For this review, take the finished solid that the model builds, in its own axes (mm). Face numbers are marked on the shaded views. A direction names the side the tool comes from. Round coordinates to 2 decimals unless told otherwise and drop trailing zeros. Loops run counter-clockwise (first coordinate to the right, second up) from the corner with the lowest first, then second, coordinate; pieces in that order, holes last.
1. Clearance check with flat-ended pins moving along their axes: pin 1 Ø2 at (x, z) = (8.5, 10.5) entering from -Y; pin 2 Ø1 at (y, z) = (-14, 14.5) entering from -X; pin 3 Ø4 at (x, z) = (-12.5, 13) entering from +Y. State where each tip first meets the part, or that it passes through.
2. Tool access review of the marked faces 1, 2 and 3: name each direction out of +Z, -Z, +X, -X, +Y, -Y from which nothing blocks a thin tool from reaching the whole face with its end or side.
3. Consider section C-C on z = 3. State the section outline as (x, y) points, then the cut area to 3 significant figures.
4. Consider section B-B on x = 23.5. State the section outline as (y, z) points, then the cut area to 3 significant figures.
5. Draft analysis for pull direction Y (two halves, no side actions). For the marked faces 4, 5, 6 and 7, state which applies: released by +Y, released by -Y, zero draft, split by the parting line, or undercut.
6. Consider section D-D on x = -8. State the section outline as (y, z) points, then the cut area to 3 significant figures.
7. To check wall thickness, follow line 1 along Y through (x, z) = (-23.5, 3.85); line 2 along Y through (x, z) = (0, 8); line 3 along Z through (x, y) = (-17.5, -22). State the ranges of each line that lie inside material, in increasing order.
8. Consider section A-A on y = 0. State the section outline as (x, z) points.
from build123d import *

# Parameters (mm, degrees)
SKETCH1_W           = 53
SKETCH1_H           = 49
BOSS_EXTRUDE1_DEPTH = 5
SKETCH2_R           = 24.5
BOSS_EXTRUDE2_DEPTH = 16
SKETCH4_R           = 1.6
CUT_EXTRUDE1_DEPTH  = 22
SKETCH5_R           = 18.6
CUT_EXTRUDE2_DEPTH  = 7
SKETCH6_R           = 16.5
CUT_EXTRUDE3_DEPTH  = 15


with BuildPart() as part:
    # Sketch1 → Boss-Extrude1 (new body)
    with BuildSketch(Plane.XY):
        Rectangle(SKETCH1_W, SKETCH1_H)
    extrude(amount=BOSS_EXTRUDE1_DEPTH)

    # Sketch2 → Boss-Extrude2 (add)
    with BuildSketch(Plane.XY.offset(5)):
        Circle(SKETCH2_R)
    extrude(amount=BOSS_EXTRUDE2_DEPTH)

    # Sketch4 → Cut-Extrude1 (cut, through all)
    with BuildSketch(Plane(origin=(0, 0, 0), x_dir=(-1, 0, 0), z_dir=(0, 0, -1))):
        with Locations((23.5, -21.5)):
            Circle(SKETCH4_R)
        with Locations((-23.5, -21.5)):
            Circle(SKETCH4_R)
        with Locations((23.5, 21.5)):
            Circle(SKETCH4_R)
        with Locations((-23.5, 21.5)):
            Circle(SKETCH4_R)
    extrude(amount=-CUT_EXTRUDE1_DEPTH, mode=Mode.SUBTRACT)

    # Sketch5 → Cut-Extrude2 (cut)
    with BuildSketch(Plane.XY.offset(21)):
        Circle(SKETCH5_R)
    extrude(amount=-CUT_EXTRUDE2_DEPTH, mode=Mode.SUBTRACT)

    # Sketch6 → Cut-Extrude3 (cut, through all)
    with BuildSketch(Plane.XY.offset(14)):
        Circle(SKETCH6_R)
    extrude(amount=-CUT_EXTRUDE3_DEPTH, mode=Mode.SUBTRACT)


solid = part.part
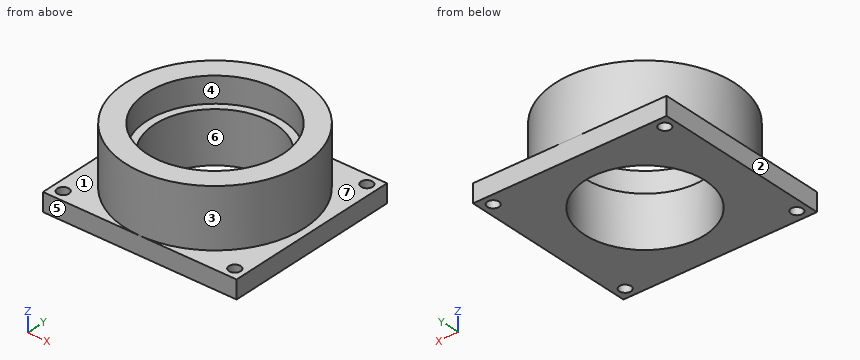
Resolved:
1. pin 1: stops at y = -23.32
1. pin 2: stops at x = -20.45
1. pin 3: stops at y = 22.14
2. face 1: +Z, -X
2. face 2: +Z, -Z, -X, +Y, -Y
2. face 3: +Z
3. outline: (-26.5, -24.5) - (26.5, -24.5) - (26.5, 24.5) - (-26.5, 24.5) - close; hole circle Ø3.2 at (-23.5, -21.5); hole circle Ø3.2 at (-23.5, 21.5); hole circle Ø33 at (0, 0); hole circle Ø3.2 at (23.5, -21.5); hole circle Ø3.2 at (23.5, 21.5)
3. area: 1,710 mm2
4. outline: (-24.5, 0) - (-23.1, 0) - (-23.1, 5) - (-24.5, 5) - close; (-19.9, 0) - (19.9, 0) - (19.9, 5) - (6.93, 5) - (6.93, 21) - (-6.93, 21) - (-6.93, 5) - (-19.9, 5) - close; (23.1, 0) - (24.5, 0) - (24.5, 5) - (23.1, 5) - close
4. area: 435 mm2
5. face 4: undercut
5. face 5: released by -Y
5. face 6: undercut
5. face 7: zero draft
6. outline: (-24.5, 0) - (-14.43, 0) - (-14.43, 14) - (-16.79, 14) - (-16.79, 21) - (-23.16, 21) - (-23.16, 5) - (-24.5, 5) - close; (14.43, 0) - (24.5, 0) - (24.5, 5) - (23.16, 5) - (23.16, 21) - (16.79, 21) - (16.79, 14) - (14.43, 14) - close
6. area: 347 mm2
7. line 1: y = -24.5 to -23.1, -19.9 to 19.9, 23.1 to 24.5
7. line 2: y = -24.5 to -16.5, 16.5 to 24.5
7. line 3: z = 0 to 5
8. outline: (-26.5, 0) - (-16.5, 0) - (-16.5, 14) - (-18.6, 14) - (-18.6, 21) - (-24.5, 21) - (-24.5, 5) - (-26.5, 5) - close; (16.5, 0) - (26.5, 0) - (26.5, 5) - (24.5, 5) - (24.5, 21) - (18.6, 21) - (18.6, 14) - (16.5, 14) - close
